from build123d import *

# Parameters (mm, degrees)
BOSS_EXTRUDE1_DEPTH = 35
SKETCH2_R           = 15
CUT_EXTRUDE1_DEPTH  = 58.786414072
SKETCH6_OUTSIDE_W   = 110.956
SKETCH6_OUTSIDE_H   = 102.162
SKETCH6_OUTSIDE_R   = 29.714468975
CUT_EXTRUDE5_DEPTH  = 10
CUT_EXTRUDE5_DRAFT  = -45


with BuildPart() as part:
    # Sketch1 → Boss-Extrude1 (new body)
    with BuildSketch(Plane(origin=(0, 0, 0), x_dir=(1, 0, 0), z_dir=(0, 1, 0))):
        Polygon((17.741058042, -29.753232758), (34.637584434, 0.487590575), (16.896526392, 30.240823333), (-17.741058042, 29.753232758), (-34.637584434, -0.487590575), (-16.896526392, -30.240823333), align=None)
    extrude(amount=BOSS_EXTRUDE1_DEPTH)

    # Sketch2 → Cut-Extrude1 (cut, through all)
    with BuildSketch(Plane(origin=(0, 35, 0), x_dir=(1, 0, 0), z_dir=(0, 1, 0))):
        with Locations(Location((0, 0, 0), (0, 0, 270))):
            Circle(SKETCH2_R)
    extrude(amount=-CUT_EXTRUDE1_DEPTH, mode=Mode.SUBTRACT)


with BuildPart() as cut_extrude5_tool:
    # Sketch6 outside → Cut-Extrude5 (with draft: the straight prism first)
    with BuildSketch(Plane(origin=(0, 35, 0), x_dir=(1, 0, 0), z_dir=(0, 1, 0))):
        Rectangle(SKETCH6_OUTSIDE_W, SKETCH6_OUTSIDE_H)
        Circle(SKETCH6_OUTSIDE_R, mode=Mode.SUBTRACT)
    extrude(amount=-CUT_EXTRUDE5_DEPTH)
    # Cut-Extrude5: the draft: its side faces are tilted about the plane it starts from
    cut_extrude5_sides = [cut_extrude5_tool.faces().sort_by_distance(p)[0] for p in [
        (0, 30, 51.081),
        (55.478, 30, 0),
        (0, 30, -51.081),
        (-55.478, 30, 0),
        (-29.714468975, 30, 0),
    ]]
    draft(cut_extrude5_sides, Plane(origin=(0, 35, 0), x_dir=(1, 0, 0), z_dir=(0, 1, 0)), CUT_EXTRUDE5_DRAFT)


with BuildPart() as part_1:
    add(part.part)

    # Cut-Extrude5: cut by cut_extrude5_tool
    add(cut_extrude5_tool.part, mode=Mode.SUBTRACT)


solid = part_1.part
Here's how the part is built. I have some questions about the finished solid (model axes, mm). Give positions to 0.01 mm unless a question says otherwise; leave off trailing zeros. Order: outer loops, then holes, each group sorted by start corner. A loop starts at its lowest first (then second) coordinate and runs counter-clockwise, first axis right, second up. Notation, with made-up numbers: M 16.5,-37 L 66.5,-37 A12 ccw 66.5,-20 Z; hole C 82,-12 d2. An arc over 180 degrees is marked long. Answer as a JSON object with one key per item and string values. Group by question number.
1) Suppose I cut it at C-C, the plane y = 2. Write out the boundary of the cut face in (x, z), plus the area to 3 significant figures.
2) Please list where these lines run through material, in increasing order: L1, parallel to Z at x = 11.5, y = 8.5; L2, parallel to X at y = 16, z = 0; L3, parallel to X at y = 21.5, z = -13. Write a range as [from, to].
3) Suppose I cut it at A-A, the plane x = 0. Write out the boundary of the cut face in (y, z), plus the area to 3 significant figures.
4) Suppose I cut it at B-B, the plane y = 32.5. Write out the boundary of the cut face in (x, z), plus the area to 3 significant figures.
5) I'm going to push flat-ended pins straight in: pin 1 Ø24 at (x, z) = (0, 0) entering from +Y; pin 2 Ø2 at (y, z) = (5, -8) entering from +X; pin 3 Ø12 at (x, y) = (24.5, 19.5) entering from +Z; pin 4 Ø6 at (y, z) = (15, 3.5) entering from +X. Where does each tip first touch, or does it pass through?
6) We'd pull the mould along X, two halves only. Please class faces 1 (the cylindrical face through (0.66, 17.745, -14.985)), 2 (the flat face through (7, 0, -14)), 3 (the conical face through (27.67, 34.76, 11.47)): pulls with the +X half, pulls with the -X half, needs draft (parallel to the pull), parting line crosses it, or undercut.
Results found:
{
 "1": {"outline": "M -34.64,0.49 L -17.74,-29.75 L 16.9,-30.24 L 34.64,-0.49 L 17.74,29.75 L -16.9,30.24 Z; hole C 0,0 d30", "area": "2,410 mm²"},
 "2": {"L1": "[-30.16, -9.63], [9.63, 29.84]", "L2": "[-34.37, -15], [15, 34.37]", "L3": "[-27.1, -7.48], [7.48, 27.18]"},
 "3": {"outline": "M 0,-30 L 34.71,-30 L 35,-29.71 L 35,-15 L 0,-15 Z; M 0,15 L 35,15 L 35,29.71 L 34.71,30 L 0,30 Z", "area": "1,050 mm²"},
 "4": {"outline": "M -31.91,-4.39 L -20.46,-24.88 A32.21 ccw -12.16,-29.83 L 11.31,-30.16 A32.21 ccw 19.76,-25.45 L 31.78,-5.28 A32.21 ccw 31.91,4.39 L 20.46,24.88 A32.21 ccw 12.16,29.83 L -11.31,30.16 A32.21 ccw -19.76,25.45 L -31.78,5.28 A32.21 ccw Z; hole C 0,0 d30", "area": "2,340 mm²"},
 "5": {"pin 1": "through", "pin 2": "x = 30.75", "pin 3": "z = 28.39", "pin 4": "x = 34.09"},
 "6": {"face 1": "undercut", "face 2": "needs draft", "face 3": "parting line crosses it"}
}
